Can you work these out from the model? Positions are in its coordinate system, mm. A direction names the side the tool comes from. Give positions to 0.01 mm unless a question says otherwise; leave off trailing zeros. Write each loop counter-clockwise with the first axis right and the second up, starting at its lowest first coordinate (ties: lowest second). Pieces come first, ordered by that corner, then holes. Notation, with made-up numbers: M -38,63 L -10,63 A16 ccw -10,69 Z; hole C 31,22.25 d4. An arc over 180 degrees is marked long. Write each question's results on one line, items separated by ' | '.
from build123d import *

# Parameters (mm, degrees)
SKETCH_1_W          = 56.5
SKETCH_1_H          = 25.2
EXTRUDE_1_DEPTH     = 19
SKETCH_2_W          = 56.5
SKETCH_2_H          = 25.2
EXTRUDE_2_DEPTH     = 2.5
SKETCH_3_W          = 34.2
SKETCH_3_H          = 12.4
EXTRUDE_3_DEPTH     = 1
CUT_EXTRUDE_1_DEPTH = 1.8
SKETCH_5_W          = 54
SKETCH_5_H          = 22.2
CUT_EXTRUDE_2_DEPTH = 1.2
CUT_EXTRUDE_3_DEPTH = 4.2
FILLET_1_R          = 3
FILLET_2_R          = 3
SKETCH_8_R          = 1.3
CUT_EXTRUDE_4_DEPTH = 4.2
SKETCH_9_R          = 2.6
CUT_EXTRUDE_5_DEPTH = 1.5
SKETCH_10_R         = 0.5
CUT_EXTRUDE_6_DEPTH = 4


with BuildPart() as part:
    # Эскиз1 → Бобышка-Вытянуть1 (new body)
    with BuildSketch(Plane.XY):
        with Locations((-22.317513824, -999.289755901)):
            Rectangle(SKETCH_1_W, SKETCH_1_H)
        Polygon((-48.767513824, -989.189755901), (3.432486176, -989.189755901), (3.432486176, -1009.389755901), (-48.767513824, -1009.389755901), (-48.767513824, -996.989755901), (-14.567513824, -996.989755901), (-14.567513824, -1002.989755901), (-13.767513824, -1002.989755901), (-13.767513824, -996.989755901), (-13.767513824, -996.389755901), (-48.767513824, -996.389755901), align=None, mode=Mode.SUBTRACT)
    extrude(amount=EXTRUDE_1_DEPTH)

    # Эскиз2 → Бобышка-Вытянуть2 (add)
    with BuildSketch(Plane(origin=(0, 0, 0), x_dir=(-1, 0, 0), z_dir=(0, 0, -1))):
        with Locations((22.317513824, -999.289755901)):
            Rectangle(SKETCH_2_W, SKETCH_2_H)
    extrude(amount=EXTRUDE_2_DEPTH)

    # Эскиз3 → Бобышка-Вытянуть3 (add)
    with BuildSketch(Plane.XY):
        with Locations((-31.667513824, -1003.189755901)):
            Rectangle(SKETCH_3_W, SKETCH_3_H)
    extrude(amount=EXTRUDE_3_DEPTH)

    # Эскиз4 → Вырез-Вытянуть1 (cut)
    with BuildSketch(Plane.ZY.offset(50.567513824)):
        with BuildLine():
            Line((14.666630398, -1000.489317936), (14.666630398, -999.889317936))
            ThreePointArc((14.666630398, -999.889317936), (14.233148434, -998.8427999), (13.186630398, -998.409317936))
            Line((13.186630398, -998.409317936), (6.806630398, -998.409317936))
            ThreePointArc((6.806630398, -998.409317936), (5.760112362, -998.8427999), (5.326630398, -999.889317936))
            Line((5.326630398, -999.889317936), (5.326630398, -1000.489317936))
            ThreePointArc((5.326630398, -1000.489317936), (5.760112362, -1001.535835972), (6.806630398, -1001.969317936))
            Line((6.806630398, -1001.969317936), (13.186630398, -1001.969317936))
            ThreePointArc((13.186630398, -1001.969317936), (14.233148434, -1001.535835972), (14.666630398, -1000.489317936))
        make_face()
    extrude(amount=-CUT_EXTRUDE_1_DEPTH, mode=Mode.SUBTRACT)

    # Эскиз5 → Вырез-Вытянуть2 (cut)
    with BuildSketch(Plane.XY.offset(19)):
        with Locations((-22.567513824, -999.289755901)):
            Rectangle(SKETCH_5_W, SKETCH_5_H)
    extrude(amount=-CUT_EXTRUDE_2_DEPTH, mode=Mode.SUBTRACT)

    # Эскиз7 → Вырез-Вытянуть3 (cut)
    with BuildSketch(Plane(origin=(5.932486176, 0, 0), x_dir=(0, 0, -1), z_dir=(1, 0, 0))):
        with BuildLine():
            Line((-12.15, -1001.486817264), (-12.15, -1004.892694537))
            ThreePointArc((-12.15, -1004.892694537), (-6.35, -1003.189755901), (-12.15, -1001.486817264))
        make_face()
    extrude(amount=-CUT_EXTRUDE_3_DEPTH, mode=Mode.SUBTRACT)

    # Скругление1
    fillet_1_edges = [part.edges().sort_by_distance(p)[0] for p in [
        (5.932486176, -999.289755901, -2.5),
        (-22.317513824, -1011.889755901, -2.5),
        (-50.567513824, -999.289755901, -2.5),
        (-22.317513824, -986.689755901, -2.5),
    ]]
    fillet(fillet_1_edges, radius=FILLET_1_R)

    # Скругление2
    # the kernel refuses this fillet: 3 mm, written as the material it takes off along each edge
    with BuildSketch(Plane(origin=(-47.567513824, -1008.889755901, 0.5), x_dir=(0, -1, 0), z_dir=(-1, 0, 0))) as fillet_2_piece_1_section:
        Polygon((0, 0), (FILLET_2_R, 0), (FILLET_2_R, -FILLET_2_R), (0, -FILLET_2_R), align=None)
    fillet_2_piece_1 = extrude(amount=FILLET_2_R, mode=Mode.PRIVATE)
    fillet_2_piece_1 = fillet_2_piece_1 - Plane(origin=(-47.567513824, -1008.889755901, 0.5), x_dir=(0, 0.7071067811865475, 0.7071067811865475), z_dir=(-1, 0, 0)) * Sphere(FILLET_2_R, mode=Mode.PRIVATE)
    add(fillet_2_piece_1, mode=Mode.SUBTRACT)
    with BuildSketch(Plane(origin=(2.932486176, -1008.889755901, 0.5), x_dir=(0, -1, 0), z_dir=(1, 0, 0))) as fillet_2_piece_2_section:
        Polygon((0, 0), (FILLET_2_R, 0), (FILLET_2_R, FILLET_2_R), (0, FILLET_2_R), align=None)
    fillet_2_piece_2 = extrude(amount=FILLET_2_R, mode=Mode.PRIVATE)
    fillet_2_piece_2 = fillet_2_piece_2 - Plane(origin=(2.932486176, -1008.889755901, 0.5), x_dir=(0, 0.7071067811865475, 0.7071067811865475), z_dir=(1, 0, 0)) * Sphere(FILLET_2_R, mode=Mode.PRIVATE)
    add(fillet_2_piece_2, mode=Mode.SUBTRACT)
    with BuildSketch(Plane(origin=(-47.567513824, -989.689755901, 0.5), x_dir=(-1, 0, 0), z_dir=(0, 1, 0))) as fillet_2_piece_3_section:
        Polygon((0, 0), (FILLET_2_R, 0), (FILLET_2_R, -FILLET_2_R), (0, -FILLET_2_R), align=None)
    fillet_2_piece_3 = extrude(amount=FILLET_2_R, mode=Mode.PRIVATE)
    fillet_2_piece_3 = fillet_2_piece_3 - Plane(origin=(-47.567513824, -989.689755901, 0.5), x_dir=(0.7071067811865475, 0, 0.7071067811865475), z_dir=(0, 1, 0)) * Sphere(FILLET_2_R, mode=Mode.PRIVATE)
    add(fillet_2_piece_3, mode=Mode.SUBTRACT)
    with BuildSketch(Plane(origin=(2.932486176, -989.689755901, 0.5), x_dir=(1, 0, 0), z_dir=(0, 1, 0))) as fillet_2_piece_4_section:
        Polygon((0, 0), (FILLET_2_R, 0), (FILLET_2_R, FILLET_2_R), (0, FILLET_2_R), align=None)
    fillet_2_piece_4 = extrude(amount=FILLET_2_R, mode=Mode.PRIVATE)
    fillet_2_piece_4 = fillet_2_piece_4 - Plane(origin=(2.932486176, -989.689755901, 0.5), x_dir=(-0.7071067811865475, 0, 0.7071067811865475), z_dir=(0, 1, 0)) * Sphere(FILLET_2_R, mode=Mode.PRIVATE)
    add(fillet_2_piece_4, mode=Mode.SUBTRACT)
    with BuildSketch(Plane(origin=(-50.567513824, -986.689755901, 0.5), x_dir=(1, 0, 0), z_dir=(0, 0, 1)), Plane(origin=(5.932486176, -986.689755901, 26.5), x_dir=(-1, 0, 0), z_dir=(0, 0, -1)), Plane(origin=(5.932486176, -1011.889755901, 26.5), x_dir=(0, 1, 0), z_dir=(0, 0, -1)), Plane(origin=(-50.567513824, -1011.889755901, 0.5), x_dir=(0, 1, 0), z_dir=(0, 0, 1))) as fillet_2_piece_5:
        with BuildLine():
            CenterArc((FILLET_2_R, -FILLET_2_R), FILLET_2_R, 90, 90)
            Line((0, -FILLET_2_R), (0, 0))
            Line((0, 0), (FILLET_2_R, 0))
        make_face()
    extrude(amount=26, mode=Mode.SUBTRACT)

    # Эскиз8 → Вырез-Вытянуть4 (cut)
    with BuildSketch(Plane.XZ.offset(1011.889755901)):
        with Locations(Location((-45.267513824, 5.8, 0), (0, 0, 270))):
            Circle(SKETCH_8_R)
        with Locations(Location((-45.267513824, 13.3, 0), (0, 0, 270))):
            Circle(SKETCH_8_R)
    extrude(amount=-CUT_EXTRUDE_4_DEPTH, mode=Mode.SUBTRACT)

    # Эскиз9 → Вырез-Вытянуть5 (cut)
    with BuildSketch(Plane(origin=(0, -1009.389755901, 0), x_dir=(1, 0, 0), z_dir=(0, 1, 0))):
        with Locations(Location((-45.267513824, -5.8, 0), (0, 0, 270))):
            Circle(SKETCH_9_R)
        with Locations(Location((-45.267513824, -13.3, 0), (0, 0, 270))):
            Circle(SKETCH_9_R)
    extrude(amount=-CUT_EXTRUDE_5_DEPTH, mode=Mode.SUBTRACT)

    # Эскиз10 → Вырез-Вытянуть6 (cut)
    with BuildSketch(Plane.XZ.offset(1011.889755901)):
        with Locations(Location((-40.767513824, 4.8, 0), (0, 0, 270))):
            Circle(SKETCH_10_R)
        with Locations(Location((-40.767513824, 14.8, 0), (0, 0, 270))):
            Circle(SKETCH_10_R)
    extrude(amount=-CUT_EXTRUDE_6_DEPTH, mode=Mode.SUBTRACT)


solid = part.part
Item 1: I want a section at D-D, the plane y = -992.75. Please give me the cut outline in (x, z), and give its area (3 significant figures).
Geometry says:
outline: M -50.57,0.5 A3 ccw -47.57,-2.5 L 2.93,-2.5 A3 ccw 5.93,0.5 L 5.93,19 L 4.43,19 L 4.43,17.8 L 3.43,17.8 L 3.43,0 L -48.77,0 L -48.77,17.8 L -49.57,17.8 L -49.57,19 L -50.57,19 Z | area: 217 mm2
Item 2: I want a section at B-B, the plane z = 1.75. Please give me the cut outline in (x, y).
Geometry says:
outline: M -50.57,-1008.89 A3 ccw -47.57,-1011.89 L 2.93,-1011.89 A3 ccw 5.93,-1008.89 L 5.93,-989.69 A3 ccw 2.93,-986.69 L -47.57,-986.69 A3 ccw -50.57,-989.69 Z; hole M -48.77,-1009.39 L 3.43,-1009.39 L 3.43,-989.19 L -48.77,-989.19 L -48.77,-996.39 L -13.77,-996.39 L -13.77,-1002.99 L -14.57,-1002.99 L -14.57,-996.99 L -48.77,-996.99 Z
Item 3: I'm going to push flat-ended pins straight in: pin 1 (3.5 mm diameter, centred on y = -1003.5, z = 10, fed in from +X); pin 2 (1.5 mm diameter, centred on x = -6.5, y = -1006, fed in from +Z); pin 3 (2 mm diameter, centred on x = -50, z = 10, fed in from +Y). Where does each tip first touch, or does it pass through?
Geometry says:
pin 1: stops at x = -13.77 | pin 2: stops at z = 0 | pin 3: stops at y = -987.05
Item 4: If I drill on line 1 (X direction, y = -999, z = 15.5); line 2 (Y direction, x = -14.5, z = 5); line 3 (Y direction, x = -27.5, z = 4), over which ranges is the centre line in solid material (lowest first)? Write a range as from..to.
Geometry says:
line 1: x = -50.57..-48.77, -14.57..-13.77, 3.43..5.93 | line 2: y = -1011.89..-1009.39, -1002.99..-996.39, -989.19..-986.69 | line 3: y = -1011.89..-1009.39, -996.99..-996.39, -989.19..-986.69
Item 5: For faces 3 (the face through (5, -1003, 12.15)), 4 (the face through (-23, -989.19, 9)), 5 (the face through (-49.68, -1001.55, 14.22)), 6 (the face through (-46, -1010.89, 12)), 7 (the face through (-40.346, -1010.657, 14.531)), which set-ups out of +Z, -Z, +X, -X, +Y, -Y let a thin tool reach every point of the face, with its end or its side?
Geometry says:
face 3: +X | face 4: +Z | face 5: -X | face 6: none | face 7: -Y
Item 6: I want a section at A-A, the plane z = 9.5. Please give me the cut outline in (x, y).
Geometry says:
outline: M -50.57,-1008.89 A3 ccw -47.57,-1011.89 L 2.93,-1011.89 A3 ccw 5.93,-1008.89 L 5.93,-1006.34 L 3.43,-1006.34 L 3.43,-1009.39 L -48.77,-1009.39 L -48.77,-1001.97 L -50.57,-1001.97 Z; M -50.57,-998.41 L -48.77,-998.41 L -48.77,-996.99 L -14.57,-996.99 L -14.57,-1002.99 L -13.77,-1002.99 L -13.77,-996.39 L -48.77,-996.39 L -48.77,-989.19 L 3.43,-989.19 L 3.43,-1000.04 L 5.93,-1000.04 L 5.93,-989.69 A3 ccw 2.93,-986.69 L -47.57,-986.69 A3 ccw -50.57,-989.69 Z
Item 7: Thinking about a two-plate mould opening in Y: for faces 1 (the face through (-44.17, -1011.4, 12.6)), 2 (the face through (-24.7, -996.8, 17.8)), which applies, +Y half, -Y half, draft (parallel to the pull), parting line (faces both ways), or undercut?
Geometry says:
face 1: draft | face 2: undercut
Item 8: I want a section at C-C, the plane x = 0. Please give me the cut outline in (y, z), and give its area (3 significant figures).
Geometry says:
outline: M -1011.89,0.5 A3 ccw -1008.89,-2.5 L -989.69,-2.5 A3 ccw -986.69,0.5 L -986.69,19 L -988.19,19 L -988.19,17.8 L -989.19,17.8 L -989.19,0 L -1009.39,0 L -1009.39,17.8 L -1010.39,17.8 L -1010.39,19 L -1011.89,19 Z | area: 152 mm2
